Input: part model. Units: mm. Frame: model coordinates. Face numbers are marked on the shaded views. A direction names the side the tool comes from. Give positions to 0.01 mm unless a question says otherwise; leave off trailing zeros. Loops run counter-clockwise (first coordinate to the right, second up) from the corner with the lowest first, then second, coordinate; pieces in that order, holes last. Notation, with made-up numbers: (30.25, 20.5) -> (68.25, 20.5) arc R22 ccw to (68.25, 50.5) -> close; hole circle Ø4 at (-27.5, -3). An arc over 180 degrees is marked (long way). Answer as a JSON object with one key per item and string values.
```python
from build123d import *

# Parameters (mm, degrees)
F0_W     = 50.8
F0_H     = 50.8
F1_DEPTH = 6.35
F2_W     = 12.7
F2_H     = 12.7
F3_DEPTH = 101.6
F4_R     = 3.175
F5_DEPTH = 31.75
F7_DEPTH = 25.4


with BuildPart() as f1:
    # F0 (on Top) → F1 (new body)
    with BuildSketch(Plane.XY):
        with Locations((-0.287808, -0.096031)):
            Rectangle(F0_W, F0_H)
    extrude(amount=F1_DEPTH)

    # F2 (on face) → F3 (join)
    with BuildSketch(Plane.XY.offset(6.35)):
        with Locations((-0.287808, -0.096031)):
            Rectangle(F2_W, F2_H)
    extrude(amount=F3_DEPTH)

    # F4 (on face) → F5 (join)
    with BuildSketch(Plane.YZ.offset(6.062192)):
        with Locations((-0.096031, 101.6)):
            Circle(F4_R)
    extrude(amount=F5_DEPTH)

    # F6 (on face) → F7 (cut)
    with BuildSketch(Plane.XY.offset(6.35)):
        Polygon((-6.637808, -6.446031), (-6.637808, 6.253969), (-6.637808, 25.303969), (-25.687808, 25.303969), (-25.687808, -25.496031), (-6.637808, -25.496031), align=None)
    extrude(amount=-F7_DEPTH, mode=Mode.SUBTRACT)


solid = f1.part
```
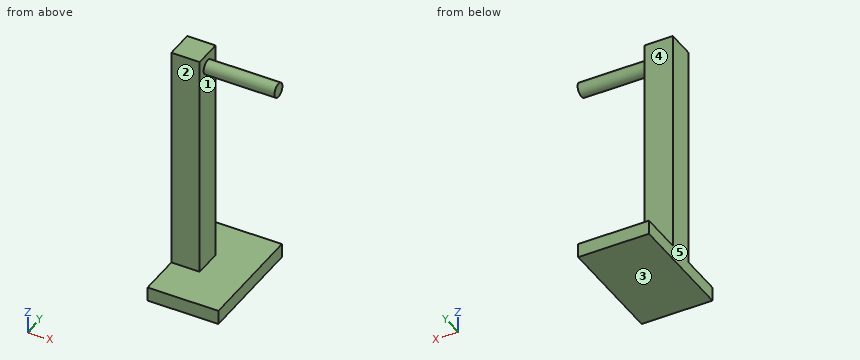
Q1. Section D-D, the plane y = -1.5. Return the cut outline in (x, z), then the cut area to 3 significant figures.
Evaluation:
{"outline": "(-6.64, 0) -> (25.11, 0) -> (25.11, 6.35) -> (6.06, 6.35) -> (6.06, 98.75) -> (37.81, 98.75) -> (37.81, 104.45) -> (6.06, 104.45) -> (6.06, 107.95) -> (-6.64, 107.95) -> close", "area": "1,670 mm2"}
Q2. Section C-C, the plane x = -3. Return the cut outline in (y, z), then the cut area to 3 significant figures.
Evaluation:
{"outline": "(-25.5, 0) -> (25.3, 0) -> (25.3, 6.35) -> (6.25, 6.35) -> (6.25, 107.95) -> (-6.45, 107.95) -> (-6.45, 6.35) -> (-25.5, 6.35) -> close", "area": "1,610 mm2"}
Q3. Access query for the marked faces 4 and 5. Directions: +Z, -Z, +X, -X, +Y, -Y. A direction counts if a zero-diameter tool reaches every point of the face in a straight line with its end or side. Return the directions, or none.
Evaluation:
{"face 4": "+Z, +X, -X, +Y", "face 5": "+Z, -Z, -X, +Y, -Y"}
Q4. Pin query (flat end, axial travel): pin 1 (4 mm diameter, centred on x = -1.5, z = 37, fed in from +Y); pin 2 (14 mm diameter, centred on y = 3, z = 39, fed in from +X); pin 3 (12 mm diameter, centred on x = 18, y = -19.5, fed in from +Z); pin 4 (5 mm diameter, centred on x = 25, y = -14, fed in from -Z). Return the tip coordinate at first contact, or that it passes through.
Evaluation:
{"pin 1": "stops at y = 6.25", "pin 2": "stops at x = 6.06", "pin 3": "stops at z = 6.35", "pin 4": "stops at z = 0"}
Q5. Section A-A, the plane x = 23. Return the cut outline in (y, z) (3 decimals).
Evaluation:
{"outline": "(-25.496, 0) -> (25.304, 0) -> (25.304, 6.35) -> (-25.496, 6.35) -> close; circle Ø6.35 at (-0.096, 101.6)"}
Q6. Draft query along Z for the marked faces 1, 2 and 3. Return one class per face: +Z half, -Z half, draft (parallel to the pull), parting line (faces both ways), or undercut.
Evaluation:
{"face 1": "undercut", "face 2": "draft", "face 3": "-Z half"}
Q7. Ray query, line 1 along Z through (x, y) = (14, -15.5); line 2 along X through (y, z) = (0.5, 23); line 3 along Z through (x, y) = (18.5, -3). Return the intervals inside material, ascending.
Evaluation:
{"line 1": "z = 0 to 6.35", "line 2": "x = -6.64 to 6.06", "line 3": "z = 0 to 6.35, 100.32 to 102.88"}
Q8. Section B-B, the plane z = 101.6. Return the cut outline in (x, y), then the cut area to 3 significant figures.
Evaluation:
{"outline": "(-6.64, -6.45) -> (6.06, -6.45) -> (6.06, -3.27) -> (37.81, -3.27) -> (37.81, 3.08) -> (6.06, 3.08) -> (6.06, 6.25) -> (-6.64, 6.25) -> close", "area": "363 mm2"}
